Autodesk Inventor part; units mm, degrees
ref_plane "YZ Plane" through (0, 0, 0) normal (1, 0, 0) x (0, 1, 0)
ref_plane "XZ Plane" through (0, 0, 0) normal (0, 1, 0) x (-1, 0, 0)
ref_plane "XY Plane" through (0, 0, 0) normal (0, 0, 1) x (1, 0, 0)
sketch "Szkic1" plane through (0, 0, 0) normal (0, 0, 1) x (1, 0, 0)
  line L0 (-144, 100) -> (144, 100)
  line L1 (144, 100) -> (144, -100)
  line L2 (144, -100) -> (-144, -100)
  line L3 (-144, -100) -> (-144, 100)
  line L4 (-144, 100) -> (144, -100) construction
  line L5 (144, 100) -> (-144, -100) construction
  point P0 (0, 0)
  dimension "d0" = 288
  dimension "d1" = 200
extrude "Wyciągnięcie proste1" add sketch "Szkic1" along normal mid plane 4
sketch "Szkic2" plane through (0, 0, 2) normal (0, 0, 1) x (1, 0, 0)
  line L0 (70, -50) -> (-70, -50)
  line L1 (-70, -50) -> (-70, 50)
  line L2 (-70, 50) -> (70, 50)
  line L3 (70, 50) -> (70, -50)
  line L4 (70, -50) -> (-70, 50) construction
  line L5 (-70, -50) -> (70, 50) construction
  line L6 (-2, 50) -> (2, 50)
  line L7 (2, 50) -> (2, -50)
  line L8 (2, -50) -> (-2, -50)
  line L9 (-2, -50) -> (-2, 50)
  line L10 (-70, 2) -> (70, 2)
  line L11 (70, 2) -> (70, -2)
  line L12 (70, -2) -> (-70, -2)
  line L13 (-70, -2) -> (-70, 2)
  line L14 (144, -100) -> (144, 100)
  line L15 (144, 95) -> (139, 95)
  line L16 (139, 95) -> (139, 83)
  line L17 (139, 83) -> (144, 83)
  line L18 (144, 83) -> (144, 95)
  line L19 (144, 100) -> (-144, 100)
  point P0 (0, 0)
  point P1 (2, -2)
  point P2 (-2, -2)
  point P3 (2, 2)
  point P4 (-2, 2)
  point P5 (144, 83)
  dimension "d4" = 140
  dimension "d5" = 100
  dimension "d6" = 4
  dimension "d7" = 100
  dimension "d8" = 68
  dimension "d9" = 4
  dimension "d10" = 48
  dimension "d13" = 5
  dimension "d14" = 12
  dimension "d15" = 5
extrude "Wyciągnięcie proste2" cut sketch "Szkic2" against normal through all contours L0 L7 L12 L3 | L0 L1 L12 L9 | L10 L7 L2 L3 | L10 L1 L2 L9
extrude "Wyciągnięcie proste3" cut sketch "Szkic2" against normal through all contours L17 L16 L15 L14
properties part number "LeftWall_Window"
Geometry: final body of the model. Coordinates: model frame, mm. Give positions to 0.01 mm unless a question says otherwise; leave off trailing zeros. Order: outer loops, then holes, each group sorted by start corner. A loop starts at its lowest first (then second) coordinate and runs counter-clockwise, first axis right, second up. Notation, with made-up numbers: (29, -8) -> (45, -8) arc R22 cw to (45, 18) -> close; hole circle Ø10 at (81.25, 73). An arc over 180 degrees is marked (long way). Write each question's results on one line, items separated by ' | '. Start each with the question number.
1) Section A-A (y = -35). Return loops of the section in (x, z).
2) First-contact query: pin 1 (12 mm diameter, centred on x = -61.5, y = 38.5, fed in from +Z). Flat tip, straight axial feed; report the tip coordinate or a pass-through.
3) Section B-B (x = 57.5). Return loops of the section in (y, z).
4) Line query: line 1 (Y direction, x = -8.5, z = -1.15); line 2 (X direction, y = 43, z = 1.7); line 3 (X direction, y = 88.5, z = 0.9). Output: solid intervals per line, ascending. Write a range as from..to.
5) Section C-C (z = 0.35). Return loops of the section in (x, y).
Calculated:
1) outline: (-144, -2) -> (-70, -2) -> (-70, 2) -> (-144, 2) -> close; (-2, -2) -> (2, -2) -> (2, 2) -> (-2, 2) -> close; (70, -2) -> (144, -2) -> (144, 2) -> (70, 2) -> close
2) pin 1: through
3) outline: (-100, -2) -> (-50, -2) -> (-50, 2) -> (-100, 2) -> close; (-2, -2) -> (2, -2) -> (2, 2) -> (-2, 2) -> close; (50, -2) -> (100, -2) -> (100, 2) -> (50, 2) -> close
4) line 1: -100..-50, -2..2, 50..100 | line 2: -144..-70, -2..2, 70..144 | line 3: -144..139
5) outline: (-144, -100) -> (144, -100) -> (144, 83) -> (139, 83) -> (139, 95) -> (144, 95) -> (144, 100) -> (-144, 100) -> close; hole (-70, -50) -> (-2, -50) -> (-2, -2) -> (-70, -2) -> close; hole (-70, 2) -> (-2, 2) -> (-2, 50) -> (-70, 50) -> close; hole (2, -50) -> (70, -50) -> (70, -2) -> (2, -2) -> close; hole (2, 2) -> (70, 2) -> (70, 50) -> (2, 50) -> close
